Geometry check sheet. Reference: the model listing, model coordinates, mm. A direction names the side the tool comes from. Give positions to 0.01 mm unless a question says otherwise; leave off trailing zeros. Write each loop counter-clockwise with the first axis right and the second up, starting at its lowest first coordinate (ties: lowest second). Pieces come first, ordered by that corner, then holes. Notation, with made-up numbers: M 41,26.25 L 49,26.25 A22 cw 49,64.25 Z; hole C 13.25,-31.75 d11. An arc over 180 degrees is marked long. Use one line per item in the form item = value. Start each with the question number.
Autodesk Fusion 360 part; units mm, degrees
sketch "Sketch1" plane through (0, 0, 0) normal (0, 0, 1) x (1, 0, 0)
  circle A0 centre (0, 0) radius 17.855
  circle A1 centre (0, 0) radius 6.75
  dimension "d1" = 35.71
  dimension "d2" = 13.5
extrude "Extrude1" add sketch "Sketch1" along normal blind 100
sketch "Sketch2" plane through (0, 0, 0) normal (0, 0, -1) x (1, 0, 0)
  circle A0 centre (0, 0) radius 6.75
  circle A1 centre (0, 0) radius 17.855
  circle A2 centre (0.2482, -12.264) radius 1.4
  circle A3 centre (10.5133, 5.8699) radius 1.4
  circle A4 centre (-10.3222, 5.8177) radius 1.4
  dimension "d5" = 2.8
  dimension "d6" = 2.8
  dimension "d7" = 2.8
extrude "Extrude2" cut sketch "Sketch2" against normal blind 13 contours A2 | A3 | A4
sketch "Sketch3" plane through (0, 0, 100) normal (0, 0, 1) x (1, 0, 0)
  circle A0 centre (0, 0) radius 28.439
  circle A1 centre (0, 0) radius 6.75
  circle A2 centre (0, 0) radius 17.855
extrude "Extrude3" add sketch "Sketch3" along normal blind 5 contours A0 | A2
sketch "Sketch4" plane through (0, 0, 100) normal (0, 0, -1) x (1, 0, 0)
  circle A0 centre (0, 0) radius 28.439
  circle A1 centre (0, 0) radius 17.855
  circle A2 centre (0, 23.0024) radius 1.6
  circle A3 centre (-19.9207, -11.5012) radius 1.6
  circle A4 centre (19.9207, -11.5012) radius 1.6
  dimension "d17" = 3.2
  dimension "d19" = 360
extrude "Extrude4" cut sketch "Sketch4" against normal blind 5 contours A2 | A3 | A4
(1) Sectioned sample at A-A, the plane y = 0. Record the boundary of the cut face in (x, z) (3 decimals).
(2) Tool access check on faces 5 (the cylindrical face through (1.001, 11.084, 6.409)), 6 (the cylindrical face through (21.447, 11.021, 102.465)). Record the directions out of +Z, -Z, +X, -X, +Y, -Y that give a thin tool (end or side, any length) a straight path to the whole face; none if there is none.
(3) Draft check along Y on faces 1 (the cylindrical face through (-1.46, 6.59, 51.76)), 2 (the cylindrical face through (-18.4, 11, 102.5)), 3 (the flat face through (6, -6, 105)), 4 (the cylindrical face through (27.126, -8.542, 102.465)). Enter one of: released by +Y, released by -Y, zero draft, split by the parting line, or undercut.
(4) Sectioned sample at B-B, the plane x = 0. Record the boundary of the cut face in (y, z) (3 decimals).
(5) Depth check by flat-ended pin: pin 1 (3.5 mm diameter, centred on x = 0, y = -23, fed in from -Z); pin 2 (1.4 mm diameter, centred on x = -10.5, y = -5.5, fed in from -Z); pin 3 (6 mm diameter, centred on x = 1, z = 56, fed in from -Y) (3 decimals). Enter the tip coordinate at first touch or a pass-through.
(6) Sectioned sample at C-C, the plane z = 38. Record the boundary of the cut face in (x, y) (3 decimals).
(7) Sectioned sample at D-D, the plane y = -14. Record the boundary of the cut face in (x, z), plus the area to 3 significant figures.
(8) Thickness scan on probe 1 along X at (y, z) = (-0.5, 70); probe 2 along Y at (x, z) = (0, 77) (3 decimals); probe 3 along Y at (x, z) = (-1, 9). Record the ranges inside material, lowest first. Write a range as [from, to].
Numbers:
q1.outline = M -28.439,100 L -17.855,100 L -17.855,0 L -6.75,0 L -6.75,105 L -28.439,105 Z; M 6.75,0 L 17.855,0 L 17.855,100 L 28.439,100 L 28.439,105 L 6.75,105 Z
q2.face_5 = -Z
q2.face_6 = +Z, -Z
q3.face_1 = undercut
q3.face_2 = undercut
q3.face_3 = zero draft
q3.face_4 = split by the parting line
q4.outline = M -28.439,100 L -24.602,100 L -24.602,105 L -28.439,105 Z; M -21.402,100 L -17.855,100 L -17.855,0 L -6.75,0 L -6.75,105 L -21.402,105 Z; M 6.75,0 L 10.886,0 L 10.886,13 L 13.642,13 L 13.642,0 L 17.855,0 L 17.855,100 L 28.439,100 L 28.439,105 L 6.75,105 Z
q5.pin_1 = 100
q5.pin_2 = 13
q5.pin_3 = -17.855
q6.outline = C 0,0 d35.71; hole C 0,0 d13.5
q7.outline = M -24.75,100 L -11.08,100 L -11.08,0 L 11.08,0 L 11.08,100 L 24.75,100 L 24.75,105 L -24.75,105 Z
q7.area = 2,460 mm2
q8.probe_1 = [-17.85, -6.73], [6.73, 17.85]
q8.probe_2 = [-17.855, -6.75], [6.75, 17.855]
q8.probe_3 = [-17.83, -6.68], [6.68, 11.63], [12.9, 17.83]
